Can you work these out from the model? Positions are in its coordinate system, mm. Face numbers are marked on the shaded views. Round coordinates to 2 decimals unless told otherwise and drop trailing zeros. Loops run counter-clockwise (first coordinate to the right, second up) from the corner with the lowest first, then second, coordinate; pieces in that order, holes last. Notation, with made-up numbers: M 66,-39 L 96,-39 A22 ccw 96,-11 Z; hole C 26.25,-27 d11. An arc over 180 degrees is marked long. Use a Markdown table: item, result. Add a question column.
```python
from build123d import *

# Parameters (mm, degrees)
SKETCH2_R          = 12.5
CUT_EXTRUDE1_DEPTH = 70


with BuildPart() as part:
    # Sketch1 → Revolve1 (revolve)
    with BuildSketch(Plane.XY, mode=Mode.PRIVATE) as revolve1_sk:
        with BuildLine():
            Line((15, 70), (35, 70))
            ThreePointArc((35, 70), (40, 75), (35, 80))
            add(Edge.make_bspline(
                [(5, 195), (5.717546725, 84.963174913), (35, 80)],
                knots=[0, 0, 0, 1, 1, 1], degree=2))
            ThreePointArc((5, 195), (3.535533906, 198.535533906), (0, 200))
            Line((0, 200), (0, 0))
            Line((0, 0), (20, 0))
            Line((20, 0), (15, 45))
            ThreePointArc((15, 45), (25, 55), (15, 65))
            Line((15, 65), (15, 70))
        make_face()
    revolve(revolve1_sk.sketch.rotate(Axis((0, 200, 0), (0, -1, 0)), 90), axis=Axis((0, 200, 0), (0, -1, 0)))

    # Sketch2 → Cut-Extrude1 (cut)
    with BuildSketch(Plane.XZ):
        with Locations(Location((0, 0, 0), (0, 0, 270))):
            Circle(SKETCH2_R)
    extrude(amount=-CUT_EXTRUDE1_DEPTH, mode=Mode.SUBTRACT)


solid = part.part
```
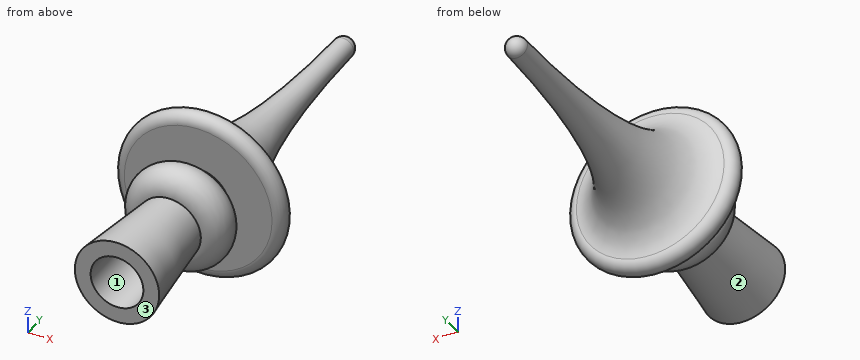
(1) Suppose I cut it at B-B on y = 73.5. List the corners of the cut face in (x, z) for me.
(2) Thinking about a two-plate mould opening in X: for the marked faces 1, 2 and 3, which applies, released by +X, released by -X, zero draft, split by the parting line, or undercut?
(3) Suppose I cut it at A-A on y = 27. List the corners of the cut face in (x, z) for me.
(4) If I drill on probe 1 along X at (y, z) = (25, 3.5); probe 2 along Y at (x, z) = (2, 22); probe 3 along Y at (x, z) = (-14, 19), over which ranges is the centre line in solid material (lowest first)? Write a range as [from, to].
(5) I'm going to push flat-ended pins straight in: pin 1 (12 mm diameter, centred on y = 92.5, z = 12, fed in from +X); pin 2 (15 mm diameter, centred on x = 0, z = 0, fed in from -Y); pin 3 (12 mm diameter, centred on x = 0, y = 93, fed in from -Z). Where does each tip first touch, or does it pass through?
Results below:
| question | item | result |
|---|---|---|
| 1 | outline | C 0,0 d79.54 |
| 2 | face 1 | undercut |
| 2 | face 2 | split by the parting line |
| 2 | face 3 | zero draft |
| 3 | outline | C 0,0 d34; hole C 0,0 d25 |
| 4 | probe 1 | x = [-16.86, -12], [12, 16.86] |
| 4 | probe 2 | y = [47.95, 62.05], [70, 89.12] |
| 4 | probe 3 | y = [49.9, 60.1], [70, 87.14] |
| 5 | pin 1 | stops at x = 21.7 |
| 5 | pin 2 | stops at y = 70 |
| 5 | pin 3 | stops at z = -23.72 |
